Source: three-view drawing plus pictorial views. Frame: mm from the lowest corner of the part. A direction names the side the tool comes from. Give positions to 0.01 mm unless a question says otherwise; leave off trailing zeros. Order: outer loops, then holes, each group sorted by start corner. A loop starts at its lowest first (then second) coordinate and runs counter-clockwise, first axis right, second up. Notation, with made-up numbers: M -21.5,-30 L -16.5,-30 A32 cw -16.5,4 Z; hole C 88.25,48 d9. An arc over 180 degrees is marked long. Use CSV: the item, a comma, the result in double quotes. Start each with the question number.
1. Section query C-C, the plane x = 142. Return the cut outline in (y, z), plus the area to 3 significant figures.
2. Line query: line 1 along X through (y, z) = (18.5, 45.5); line 2 along X through (y, z) = (37.5, 51); line 3 along Y through (x, z) = (114.5, 49). Output: solid intervals per line, ascending. Write a range as [from, to].
3. Mould query, pull axis X, two halves, no side actions, for the marked faces 1, 2, 3 and 4. Classes: released by +X, released by -X, zero draft, split by the parting line, or undercut.
4. Section query D-D, the plane y = 4. Return the cut outline in (x, z).
5. Section query A-A, the plane y = 23.5. Return the cut outline in (x, z) (3 decimals), plus the area to 3 significant figures.
6. Pin query (flat end, axial travel): P1, Ø9.5, axis at y = 6, z = 24.5, coming from the +X side; P2, Ø1.5, axis at x = 37.5, y = 12.5, coming from the -Z side (3 decimals); P3, Ø1, axis at y = 27, z = 54, coming from the +X side. Return the tip coordinate at first contact, or that it passes through.
7. Reachability of the marked faces 5, 6, 7 and 8 from +Z, -Z, +X, -X, +Y, -Y: full face, straight path, thin tool, end or side. Return the list, or none.
8. Section query B-B, the plane z = 18.5. Return the cut outline in (x, y) (3 decimals), plus the area to 3 significant figures.
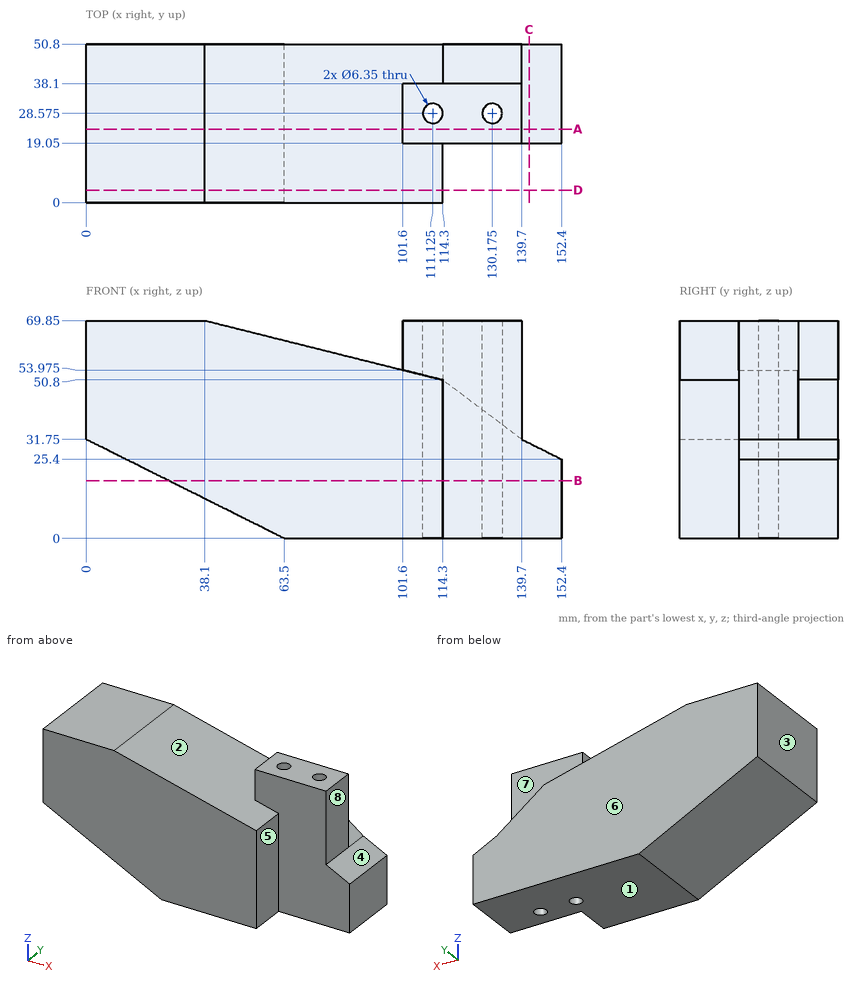
Result set:
1,outline,"M 19.05,0 L 50.8,0 L 50.8,30.6 L 19.05,30.6 Z"
1,area,"972 mm2"
2,line 1,"[0, 114.3]"
2,line 2,"[0, 139.7]"
2,line 3,"[19.05, 50.8]"
3,face 1,"zero draft"
3,face 2,"undercut"
3,face 3,"released by -X"
3,face 4,"released by +X"
4,outline,"M 0,31.75 L 63.5,0 L 114.3,0 L 114.3,50.8 L 38.1,69.85 L 0,69.85 Z"
5,outline,"M 0,31.75 L 63.5,0 L 152.4,0 L 152.4,25.4 L 139.7,31.75 L 139.7,69.85 L 101.6,69.85 L 101.6,53.975 L 38.1,69.85 L 0,69.85 Z"
5,area,"8,610 mm2"
6,P1,"x = 114.3"
6,P2,"z = 12.625"
6,P3,"x = 139.7"
7,face 5,"+Z, -Z, +X, -Y"
7,face 6,"+Z, -Z, +X, -X, +Y"
7,face 7,"+Z, +X, +Y"
7,face 8,"+Z, +X, +Y, -Y"
8,outline,"M 26.5,0 L 114.3,0 L 114.3,19.05 L 152.4,19.05 L 152.4,50.8 L 26.5,50.8 Z; hole C 111.125,28.575 d6.35; hole C 130.175,28.575 d6.35"
8,area,"5,610 mm2"
